Verification items for the finished model (mm, model axes). Face numbers are marked on the shaded views. A direction names the side the tool comes from. Round coordinates to 2 decimals unless told otherwise and drop trailing zeros. Write each loop counter-clockwise with the first axis right and the second up, starting at its lowest first coordinate (ties: lowest second). Pieces come first, ordered by that corner, then holes. Notation, with made-up numbers: (46.5, -35.75) - (56.5, -35.75) arc R37 cw to (56.5, 1.25) - close; hole circle Ø4 at (22.5, 26). An arc over 180 degrees is marked (long way). Answer as a JSON object with one key per item and string values.
```python
from build123d import *

# Parameters (mm, degrees)
F1_DEPTH = 91.44
F3_DEPTH = 38.608
F5_DEPTH = 4.7752
F6_R     = 1.35255
F7_DEPTH = 52.832


# Not quite as in the source:
# - a feature names something its author has since deleted; it is built from what else it names


with BuildPart() as f1:
    # F0 (on Top) → F1 (new body)
    with BuildSketch(Plane.XY):
        with BuildLine():
            ThreePointArc((0, 2), (0.5857864376, 0.5857864376), (2, 0))
            Line((2, 0), (105.061, 0))
            ThreePointArc((105.061, 0), (106.4752135624, 0.5857864376), (107.061, 2))
            Line((107.061, 2), (107.061, 36.1))
            ThreePointArc((107.061, 36.1), (106.4752135624, 37.5142135624), (105.061, 38.1))
            Line((105.061, 38.1), (2, 38.1))
            ThreePointArc((2, 38.1), (0.5857864376, 37.5142135624), (0, 36.1))
            Line((0, 36.1), (0, 2))
        make_face()
    extrude(amount=F1_DEPTH)

    # F2 (on face) → F3 (cut)
    with BuildSketch(Plane.XY.offset(91.44)):
        with BuildLine():
            Line((104.261, 36.3), (2.8, 36.3))
            ThreePointArc((2.8, 36.3), (2.0928932188, 36.0071067812), (1.8, 35.3))
            Line((1.8, 35.3), (1.8, 2.8))
            ThreePointArc((1.8, 2.8), (2.0928932188, 2.0928932188), (2.8, 1.8))
            Line((2.8, 1.8), (104.261, 1.8))
            ThreePointArc((104.261, 1.8), (104.9681067812, 2.0928932188), (105.261, 2.8))
            Line((105.261, 2.8), (105.261, 35.3))
            ThreePointArc((105.261, 35.3), (104.9681067812, 36.0071067812), (104.261, 36.3))
        make_face()
    extrude(amount=-F3_DEPTH, mode=Mode.SUBTRACT)

    # F4 (on face) → F5 (join)
    with BuildSketch(Plane(origin=(0, 0, 0), x_dir=(1, 0, 0), z_dir=(0, 0, -1))):
        with BuildLine():
            ThreePointArc((107.061, -2), (106.4752135624, -0.5857864376), (105.061, 0))
            Line((105.061, 0), (101.251, 0))
            Line((101.251, 0), (101.251, -2))
            ThreePointArc((101.251, -2), (102.3669231637, -4.6940768363), (105.061, -5.81))
            Line((105.061, -5.81), (107.061, -5.81))
            Line((107.061, -5.81), (107.061, -2))
        make_face()
        with BuildLine():
            Line((101.251, -36.1), (101.251, -38.1))
            Line((101.251, -38.1), (105.061, -38.1))
            ThreePointArc((105.061, -38.1), (106.4752135624, -37.5142135624), (107.061, -36.1))
            Line((107.061, -36.1), (107.061, -32.29))
            Line((107.061, -32.29), (105.061, -32.29))
            ThreePointArc((105.061, -32.29), (102.3669231637, -33.4059231637), (101.251, -36.1))
        make_face()
        with BuildLine():
            ThreePointArc((5.81, -36.1), (4.6940768363, -33.4059231637), (2, -32.29))
            Line((2, -32.29), (0, -32.29))
            Line((0, -32.29), (0, -36.1))
            ThreePointArc((0, -36.1), (0.5857864376, -37.5142135624), (2, -38.1))
            Line((2, -38.1), (5.81, -38.1))
            Line((5.81, -38.1), (5.81, -36.1))
        make_face()
        with BuildLine():
            Line((5.81, 0), (2, 0))
            ThreePointArc((2, 0), (0.5857864376, -0.5857864376), (0, -2))
            Line((0, -2), (0, -5.81))
            Line((0, -5.81), (2, -5.81))
            ThreePointArc((2, -5.81), (4.6940768363, -4.6940768363), (5.81, -2))
            Line((5.81, -2), (5.81, 0))
        make_face()
    extrude(amount=-F5_DEPTH)

    # F6 (on face) → F7 (cut, through all)
    with BuildSketch(Plane(origin=(0, 0, 0), x_dir=(1, 0, 0), z_dir=(0, 0, -1))):
        with Locations((103.8037641431, -3.2572358569)):
            Circle(F6_R)
        with Locations((3.2572358569, -3.2572358569)):
            Circle(F6_R)
        with Locations((3.2572358569, -34.8427641431)):
            Circle(F6_R)
        with Locations((103.8037641431, -34.8427641431)):
            Circle(F6_R)
    extrude(amount=-F7_DEPTH, mode=Mode.SUBTRACT)


solid = f1.part
```
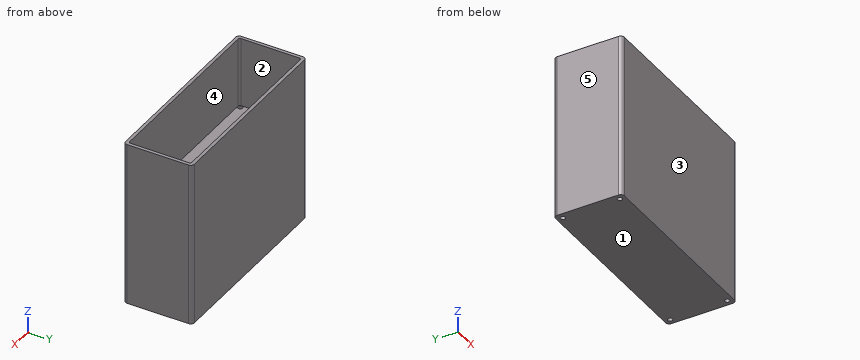
1. Access from +Z, -Z, +X, -X, +Y, -Y to the whole of each face (thin tool, end or side, straight path). Record for the marked faces 1 and 2.
Completed:
{"face 1": "-Z, +X, -X, +Y, -Y", "face 2": "+Z"}
2. Mould release check, pull along X, two halves, no side actions. Record for the marked faces 3, 4 and 5: released by +X, released by -X, zero draft, split by the parting line, or undercut.
Completed:
{"face 3": "zero draft", "face 4": "undercut", "face 5": "released by -X"}
3. Cross-section at B-B (x = 24). Record the boundary of the cut face in (y, z), plus the area to 3 significant figures.
Completed:
{"outline": "(0, 0) - (38.1, 0) - (38.1, 91.44) - (36.3, 91.44) - (36.3, 52.83) - (1.8, 52.83) - (1.8, 91.44) - (0, 91.44) - close", "area": "2,150 mm^2"}
4. Cross-section at A-A (z = 86.5). Record the boundary of the cut face in (x, y).
Completed:
{"outline": "(0, 2) arc R2 ccw to (2, 0) - (105.06, 0) arc R2 ccw to (107.06, 2) - (107.06, 36.1) arc R2 ccw to (105.06, 38.1) - (2, 38.1) arc R2 ccw to (0, 36.1) - close; hole (1.8, 2.8) arc R1 ccw to (2.8, 1.8) - (104.26, 1.8) arc R1 ccw to (105.26, 2.8) - (105.26, 35.3) arc R1 ccw to (104.26, 36.3) - (2.8, 36.3) arc R1 ccw to (1.8, 35.3) - close"}
5. Cross-section at C-C (y = 11). Record the boundary of the cut face in (x, z).
Completed:
{"outline": "(0, 0) - (107.06, 0) - (107.06, 91.44) - (105.26, 91.44) - (105.26, 52.83) - (1.8, 52.83) - (1.8, 91.44) - (0, 91.44) - close"}
6. Go/stop test with flat-tipped pins: pin 1 (10 mm diameter, centred on x = 29.5, y = 13, fed in from +Z); pin 2 (1.6 mm diameter, centred on x = 3.26, y = 34.84, fed in from -Z). Record where each tip stops, or that it passes through.
Completed:
{"pin 1": "stops at z = 52.83", "pin 2": "passes through"}
7. Material ranges on probe 1 along X at (y, z) = (15, 84.5); probe 2 along Y at (x, z) = (85.5, 59.5); probe 3 along Z at (x, y) = (26, 30), recorded low to high. Write a range as from..to.
Completed:
{"probe 1": "x = 0..1.8, 105.26..107.06", "probe 2": "y = 0..1.8, 36.3..38.1", "probe 3": "z = 0..52.83"}
